from build123d import *

# Parameters (mm, degrees)
F0_W     = 6
F0_H     = 10
F1_DEPTH = 1
F2_R     = 0.5
F7_R     = 0.25
F8_SIZE  = 0.25


with BuildPart() as f1:
    # F0 (on Top) → F1 (new body)
    with BuildSketch(Plane.XY):
        with Locations((3, 5)):
            Rectangle(F0_W, F0_H)
    extrude(amount=F1_DEPTH)

    # F2
    f2_edges = [f1.edges().sort_by_distance(p)[0] for p in [
        (6, 0, 0.5),
        (6, 10, 0.5),
        (0, 0, 0.5),
        (0, 10, 0.5),
    ]]
    fillet(f2_edges, radius=F2_R)

    # F6: sweep along a path in F5
    with BuildLine(Plane.XY.offset(1)) as f6_path:
        ThreePointArc((5.5, 0), (5.8535533906, 0.1464466094), (6, 0.5))
        Line((6, 0.5), (6, 9.5))
        ThreePointArc((6, 9.5), (5.8535533906, 9.8535533906), (5.5, 10))
        Line((5.5, 10), (0.5, 10))
        ThreePointArc((0.5, 10), (0.1464466094, 9.8535533906), (0, 9.5))
        Line((0, 9.5), (0, 0.5))
        ThreePointArc((0, 0.5), (0.1464466094, 0.1464466094), (0.5, 0))
        Line((0.5, 0), (5.5, 0))
    # F4 (on offset) → F6 (sweep)
    with BuildSketch(Plane.XZ.offset(-0.5)):
        Polygon((6, 1), (6, 0), (5.5, 0), (5.5, -0.5), (6.5, -0.5), (6.5, 1.5), (5.5, 1.5), (5.5, 1), align=None)
    sweep(path=f6_path.line)

    # F7
    f7_edges = [f1.edges().sort_by_distance(p)[0] for p in [
        (-0.5, 5, 1.5),
        (3, -0.5, -0.5),
    ]]
    fillet(f7_edges, radius=F7_R)

    # F8
    f8_edges = [f1.edges().sort_by_distance(p)[0] for p in [
        (0.5, 5, 1.5),
        (3, 9.5, 1.5),
        (5.5, 5, 1.5),
        (3, 0.5, 1.5),
        (0.5, 5, -0.5),
        (3, 0.5, -0.5),
        (5.5, 5, -0.5),
        (3, 9.5, -0.5),
    ]]
    chamfer(f8_edges, length=F8_SIZE)


solid = f1.part
Source: CAD feature listing. Evaluate the final solid. Frame: model axes, mm. Coordinates: 2 decimals unless noted, no trailing zeros. Order: outer loops, then holes, each group sorted by start corner. A loop starts at its lowest first (then second) coordinate and runs counter-clockwise, first axis right, second up. Notation, with made-up numbers: M -29.5,25.5 L -2.5,25.5 A21 cw -2.5,46.5 Z; hole C -12,21 d7. An arc over 180 degrees is marked long. Write each question's results on one line, items separated by ' | '. Start each with the question number.
1. Material intervals for L1, parallel to X at y = 3, z = 1.2; L2, parallel to Y at x = 5, z = -0.2; L3, parallel to Z at x = 4.25, y = 7, sorted ascending.
2. Draft query along Y for faces 1 (the face through (3, 5, 1)), 2 (the face through (-0.215, -0.199, 0.51)), 3 (the face through (3, 5, 0)), 4 (the face through (6.5, 5, 0)). Return one class per face: +Y half, -Y half, draft (parallel to the pull), parting line (faces both ways), or undercut.
3. Pin query (flat end, axial travel): pin 1 (2.5 mm diameter, centred on x = 3, y = 5, fed in from +Z); pin 2 (1.5 mm diameter, centred on x = 3.5, y = 6, fed in from -Z). Return the tip coordinate at first contact, or that it passes through.
4. Section B-B, the plane y = 3.25. Return the cut outline in (x, z).
5. Section A-A, the plane x = 4. Return the cut outline in (y, z), then the cut area to 3 significant figures.
Solution:
1) L1: -0.5 to 0.5, 5.5 to 6.5 | L2: -0.5 to 0.5, 9.5 to 10.5 | L3: 0 to 1
2) face 1: undercut | face 2: -Y half | face 3: undercut | face 4: draft
3) pin 1: z = 1 | pin 2: z = 0
4) outline: M -0.5,-0.25 A0.25 ccw -0.25,-0.5 L 0.25,-0.5 L 0.5,-0.25 L 0.5,0 L 5.5,0 L 5.5,-0.25 L 5.75,-0.5 L 6.25,-0.5 A0.25 ccw 6.5,-0.25 L 6.5,1.25 A0.25 ccw 6.25,1.5 L 5.75,1.5 L 5.5,1.25 L 5.5,1 L 0.5,1 L 0.5,1.25 L 0.25,1.5 L -0.25,1.5 A0.25 ccw -0.5,1.25 Z
5) outline: M -0.5,-0.25 A0.25 ccw -0.25,-0.5 L 0.25,-0.5 L 0.5,-0.25 L 0.5,0 L 9.5,0 L 9.5,-0.25 L 9.75,-0.5 L 10.25,-0.5 A0.25 ccw 10.5,-0.25 L 10.5,1.25 A0.25 ccw 10.25,1.5 L 9.75,1.5 L 9.5,1.25 L 9.5,1 L 0.5,1 L 0.5,1.25 L 0.25,1.5 L -0.25,1.5 A0.25 ccw -0.5,1.25 Z | area: 12.8 mm²
